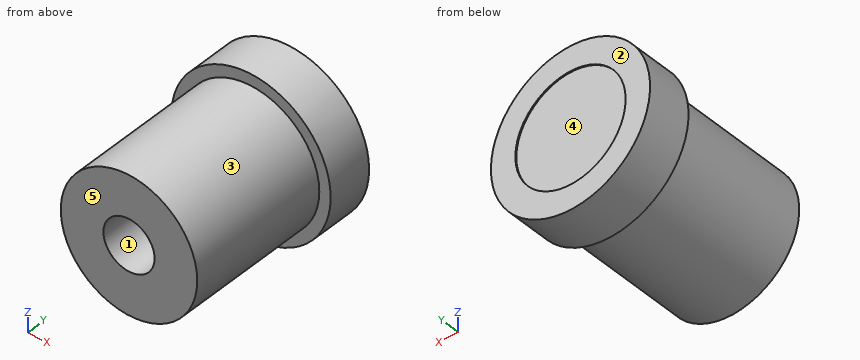
from build123d import *

# Parameters (mm, degrees)
SKETCH1_R           = 6
SKETCH1_R_2         = 2.25
BOSS_EXTRUDE1_DEPTH = 12.7
SKETCH2_R           = 7
SKETCH2_R_2         = 6
SKETCH2_R_3         = 4.85
BOSS_EXTRUDE2_DEPTH = 4
BOSS_EXTRUDE3_START = 3.9
SKETCH2_2_R         = 4.85
BOSS_EXTRUDE3_DEPTH = 0.1


with BuildPart() as part:
    # Sketch1 → Boss-Extrude1 (new body)
    with BuildSketch(Plane(origin=(0, 0, 0), x_dir=(1, 0, 0), z_dir=(0, 1, 0))):
        Circle(SKETCH1_R)
        Circle(SKETCH1_R_2, mode=Mode.SUBTRACT)
    extrude(amount=BOSS_EXTRUDE1_DEPTH)

    # Sketch2 → Boss-Extrude2 (add)
    with BuildSketch(Plane(origin=(0, 12.7, 0), x_dir=(1, 0, 0), z_dir=(0, 1, 0))):
        Circle(SKETCH2_R)
        Circle(SKETCH2_R_2, mode=Mode.SUBTRACT)
        Circle(SKETCH2_R_2)
        Circle(SKETCH2_R_3, mode=Mode.SUBTRACT)
    extrude(amount=BOSS_EXTRUDE2_DEPTH)

    # Sketch2<2> → Boss-Extrude3 (add)
    with BuildSketch(Plane(origin=(0, 12.7, 0), x_dir=(1, 0, 0), z_dir=(0, 1, 0)).offset(BOSS_EXTRUDE3_START)):
        Circle(SKETCH2_2_R)
    extrude(amount=-BOSS_EXTRUDE3_DEPTH)


solid = part.part
Part model, mm, in its own coordinate system. Face numbers are marked on the shaded views. A direction names the side the tool comes from. Give positions to 0.01 mm unless a question says otherwise; leave off trailing zeros. Write each loop counter-clockwise with the first axis right and the second up, starting at its lowest first coordinate (ties: lowest second). Pieces come first, ordered by that corner, then holes.
1) Which spindle directions (+Z, -Z, +X, -X, +Y, -Y) get a long thin tool onto all of the face, cutting with end or side? Do the marked faces 1 and 2. Say none if no direction does.
Resolved:
face 1: -Y
face 2: +Z, -Z, +X, -X, +Y
2) Cut at B-B on y = 8. Write the cut outline in (x, z).
Resolved:
outline: circle Ø12 at (0, 0); hole circle Ø4.5 at (0, 0)
3) Two-plate mould, pull along X, no slides. Class the marked faces 3, 4 and 5: released by +X, released by -X, zero draft, split by the parting line, or undercut.
Resolved:
face 3: split by the parting line
face 4: undercut
face 5: zero draft
4) Pin check, flat tips, straight feed: pin 1 (8 mm diameter, centred on x = -0.5, y = 2, fed in from +Z); pin 2 (3 mm diameter, centred on x = 2, z = -1.5, fed in from +Y); pin 3 (1.5 mm diameter, centred on x = 4.5, y = 11, fed in from +Z). Stop position of each tip, or through.
Resolved:
pin 1: stops at z = 6
pin 2: stops at y = 16.6
pin 3: stops at z = 4.68
5) Probe L1, parallel to X at y = 14.05, z = 0; L2, parallel to X at y = 4.25, z = 0; L3, parallel to Y at x = 5.25, z = -3. List the from-to ranges inside material, lowest first.
Resolved:
L1: x = -7 to -4.85, 4.85 to 7
L2: x = -6 to -2.25, 2.25 to 6
L3: y = 12.7 to 16.7
6) Cut at A-A on x = -3. Write the cut outline in (y, z), then the cut area to 3 significant figures.
Resolved:
outline: (0, -5.2) - (12.7, -5.2) - (12.7, -6.32) - (16.7, -6.32) - (16.7, -3.81) - (16.6, -3.81) - (16.6, 3.81) - (16.7, 3.81) - (16.7, 6.32) - (12.7, 6.32) - (12.7, 5.2) - (0, 5.2) - close; hole (12.7, -3.81) - (16.5, -3.81) - (16.5, 3.81) - (12.7, 3.81) - close
area: 153 mm2
7) Cut at D-D on z = 0. Write the cut outline in (x, y), then the cut area to 3 significant figures.
Resolved:
outline: (-7, 12.7) - (-6, 12.7) - (-6, 0) - (-2.25, 0) - (-2.25, 12.7) - (-4.85, 12.7) - (-4.85, 16.5) - (4.85, 16.5) - (4.85, 12.7) - (2.25, 12.7) - (2.25, 0) - (6, 0) - (6, 12.7) - (7, 12.7) - (7, 16.7) - (4.85, 16.7) - (4.85, 16.6) - (-4.85, 16.6) - (-4.85, 16.7) - (-7, 16.7) - close
area: 113 mm2
8) Cut at C-C on x = 0. Write the cut outline in (y, z), then the cut area to 3 significant figures.
Resolved:
outline: (0, -6) - (12.7, -6) - (12.7, -7) - (16.7, -7) - (16.7, -4.85) - (16.6, -4.85) - (16.6, 4.85) - (16.7, 4.85) - (16.7, 7) - (12.7, 7) - (12.7, 6) - (0, 6) - (0, 2.25) - (12.7, 2.25) - (12.7, 4.85) - (16.5, 4.85) - (16.5, -4.85) - (12.7, -4.85) - (12.7, -2.25) - (0, -2.25) - close
area: 113 mm2
